Input: part model. Units: mm. Frame: model coordinates. A direction names the side the tool comes from. Coordinates: 2 decimals unless noted, no trailing zeros. Loops run counter-clockwise (first coordinate to the right, second up) from the corner with the lowest first, then second, coordinate; pieces in that order, holes last. Notation, with made-up numbers: (52.5, 28.25) - (66.5, 28.25) arc R37 cw to (66.5, 64.25) - close; hole circle Ø1 at (26.25, 53.5). An arc over 180 degrees is marked (long way). Write item = value, one per line. Start each with the question number.
from build123d import *

# Parameters (mm, degrees)
SKETCH4_R           = 10
BOSS_EXTRUDE2_DEPTH = 6
CUT_EXTRUDE2_DEPTH  = 30


with BuildPart() as part:
    # Sketch1 → Revolve1 (revolve)
    with BuildSketch(Plane.XY):
        with BuildLine():
            Line((20.9, 0), (23.871591838, 0))
            Line((23.871591838, 0), (23.871591838, 4))
            Line((23.871591838, 4), (22.9, 4.236662843))
            Line((22.9, 4.236662843), (22.9, 51))
            ThreePointArc((22.9, 51), (22.021320344, 53.121320344), (19.9, 54))
            Line((19.9, 54), (2.764914955, 54))
            Line((2.764914955, 54), (2.764914955, 52))
            Line((2.764914955, 52), (18.9, 52))
            ThreePointArc((18.9, 52), (20.314213562, 51.414213562), (20.9, 50))
            Line((20.9, 50), (20.9, 17))
            Line((20.9, 17), (2.764914955, 17))
            Line((2.764914955, 17), (2.764914955, 15))
            Line((2.764914955, 15), (20.9, 15))
            Line((20.9, 15), (20.9, 0))
        make_face()
    revolve(axis=Axis((2.764914955, 7.821821657, 0), (0, 1, 0)))

    # Sketch4 → Boss-Extrude2 (add)
    with BuildSketch(Plane.XY.offset(22.9)):
        with Locations((1.144629865, 37)):
            Circle(SKETCH4_R)
    extrude(amount=-BOSS_EXTRUDE2_DEPTH)

    # Sketch9 → Cut-Extrude2 (cut)
    with BuildSketch(Plane(origin=(0, 54, 0), x_dir=(1, 0, 0), z_dir=(0, 1, 0))):
        with BuildLine():
            Line((-17.5, 0), (17.5, 0))
            ThreePointArc((17.5, 0), (0, 17.5), (-17.5, 0))
        make_face()
    extrude(amount=-CUT_EXTRUDE2_DEPTH, mode=Mode.SUBTRACT)


solid = part.part
Item 1: Pin query (flat end, axial travel): pin 1 (2 mm diameter, centred on x = 8, z = -9, fed in from +Y); pin 2 (10.5 mm diameter, centred on x = 5.5, y = 32.5, fed in from -Z); pin 3 (22 mm diameter, centred on x = 2.76, z = 0, fed in from -Y). Return the tip coordinate at first contact, or that it passes through.
Item 2: Cut plane C-C on y = 26. Return loops of the section in (x, z), plus the area to 3 significant figures.
Item 3: Access query for faces 4 (the flat face through (3, 15, 0)), 5 (the cylindrical face through (-7.447, 42.543, -15.836)), 6 (the flat face through (3, 17, 0)), 7 (the flat face through (-7.8, 52.4, 0)). Directions: +Z, -Z, +X, -X, +Y, -Y. A direction counts if a zero-diameter tool reaches every point of the face in a straight line with its end or side. Return the directions, or none.
Item 4: Pull-direction query (X, two-part tool) for faces 1 (the cylindrical face through (-8.846, 37.44, 20.609)), 2 (the cylindrical face through (3.24, 27.22, 17.39)), 3 (the flat face through (6, 54, 7)); classes: pulls with the +X half, pulls with the -X half, needs draft (parallel to the pull), parting line crosses it, or undercut.
Item 5: Ray query, line 1 (X direction, y = 10.5, z = 0); line 2 (Y direction, x = -4, z = 14); line 3 (Y direction, x = 14, z = -14). Return the intervals inside material, ascending.
Recorded:
q1.pin_1 = 17
q1.pin_2 = -20.14
q1.pin_3 = 15
q2.outline = (-17.37, 0) - (-15.37, 0) arc R18.14 cw (long way) to (-2.71, -17.29) arc R17.5 cw to (-16.55, -5.68) arc R20.14 ccw (long way) to start
q2.area = 208 mm²
q3.face_4 = -Y
q3.face_5 = +Y
q3.face_6 = none
q3.face_7 = -X, +Y
q4.face_1 = parting line crosses it
q4.face_2 = undercut
q4.face_3 = needs draft
q5.line_1 = -17.37 to -15.37, 20.9 to 22.9
q5.line_2 = 15 to 17, 52 to 54
q5.line_3 = 15 to 17, 50.84 to 53.89
